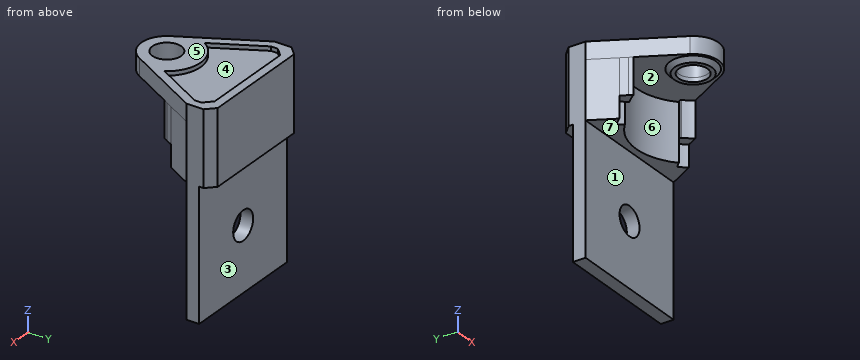
from build123d import *
from build123d.topology import SkipClean

# Parameters (mm, degrees)
BOSS_EXTRUDE1_DEPTH    = 2
BOSS_EXTRUDE2_START    = 4.75
BOSS_EXTRUDE2_DEPTH    = 4.75
BOSS_EXTRUDE3_START    = 2
SKETCH3_R              = 3
SKETCH3_R_2            = 1.7
BOSS_EXTRUDE3_DEPTH    = 2
SKETCH4_R              = 2.2
SKETCH4_R_2            = 1.7
BOSS_EXTRUDE4_DEPTH    = 0.5
CHAMFER1_SIZE          = 0.5
SKETCH5_W              = 7.5
SKETCH5_H              = 3
BOSS_EXTRUDE5_DEPTH    = 2
BOSS_EXTRUDE6_DEPTH    = 4.2
BOSS_EXTRUDE8_DEPTH    = 6.75
SKETCH10_W             = 15
SKETCH10_H             = 3
BOSS_EXTRUDE9_DEPTH    = 15.25
SKETCH11_R             = 1.65
CUT_EXTRUDE1_DEPTH     = 22.542109925
FILLET1_R              = 0.2
BOSS_EXTRUDE12_REACH   = 29.249
SKETCH16_W             = 15
SKETCH16_H             = 1.5
CUT_EXTRUDE3_DEPTH     = 0.5
CUT_EXTRUDE4_START     = -15.25
CUT_EXTRUDE4_OUTLINE_W = 15
CUT_EXTRUDE4_OUTLINE_H = 1.5
CUT_EXTRUDE4_DEPTH     = 15.25
CUT_EXTRUDE4_START_2   = -24
CUT_EXTRUDE4_2_DEPTH   = 8.75
SKETCH18_R             = 1.7
CUT_EXTRUDE5_DEPTH     = 10


# Read off the part's stored shape, not the designer's step: Cut-Extrude4
with BuildPart() as part:
    # Sketch1 → Boss-Extrude1 (new body)
    with BuildSketch(Plane.XY):
        with BuildLine():
            Line((4.594082841, 4.876925553), (5.159993549, 5.442836262))
            ThreePointArc((5.159993549, 5.442836262), (0, 7.5), (-5.159993549, 5.442836262))
            Line((-5.159993549, 5.442836262), (-4.594082841, 4.876925553))
            ThreePointArc((-4.594082841, 4.876925553), (0, 6.7), (4.594082841, 4.876925553))
        make_face()
    extrude(amount=-BOSS_EXTRUDE1_DEPTH)

    # Sketch1<3> → Boss-Extrude2 (add)
    with BuildSketch(Plane.XY.offset(BOSS_EXTRUDE2_START)):
        with BuildLine():
            Line((4.594082841, 4.876925553), (5.159993549, 5.442836262))
            ThreePointArc((5.159993549, 5.442836262), (0, 7.5), (-5.159993549, 5.442836262))
            Line((-5.159993549, 5.442836262), (-4.594082841, 4.876925553))
            ThreePointArc((-4.594082841, 4.876925553), (0, 6.7), (4.594082841, 4.876925553))
        make_face()
    extrude(amount=-BOSS_EXTRUDE2_DEPTH)

    # Sketch3 → Boss-Extrude3 (add)
    # profile 1 of 4: a face of its own
    with BuildSketch(Plane.XY.offset(4.75).offset(BOSS_EXTRUDE3_START)):
        with BuildLine():
            Line((-4.594082841, 4.876925553), (-5.159993549, 5.442836262))
            Line((-5.159993549, 5.442836262), (-2.820975701, -1.02083108))
            ThreePointArc((-2.820975701, -1.02083108), (-2.892694114, 0.795185994), (-1.902774006, 2.31936437))
            Line((-1.902774006, 2.31936437), (-2.780654635, 4.745309242))
            ThreePointArc((-2.780654635, 4.745309242), (0, 5.5), (2.780654635, 4.745309242))
            Line((2.780654635, 4.745309242), (1.902774006, 2.31936437))
            ThreePointArc((1.902774006, 2.31936437), (2.711855639, 1.282902565), (3, 0))
            ThreePointArc((3, 0), (2.954904999, -0.518205025), (2.820975701, -1.02083108))
            Line((2.820975701, -1.02083108), (5.159993549, 5.442836262))
            Line((5.159993549, 5.442836262), (4.594082841, 4.876925553))
            ThreePointArc((4.594082841, 4.876925553), (0, 6.7), (-4.594082841, 4.876925553))
        make_face()
    # profile 2 of 4: a face of its own
    with BuildSketch(Plane.XY.offset(4.75).offset(BOSS_EXTRUDE3_START)):
        with BuildLine():
            Line((-5.159993549, 5.442836262), (-4.594082841, 4.876925553))
            ThreePointArc((-4.594082841, 4.876925553), (0, 6.7), (4.594082841, 4.876925553))
            Line((4.594082841, 4.876925553), (5.159993549, 5.442836262))
            ThreePointArc((5.159993549, 5.442836262), (0, 7.5), (-5.159993549, 5.442836262))
        make_face()
    # profile 3 of 4: a face of its own
    with BuildSketch(Plane.XY.offset(4.75).offset(BOSS_EXTRUDE3_START)):
        Circle(SKETCH3_R)
        Circle(SKETCH3_R_2, mode=Mode.SUBTRACT)
    # profile 4 of 4: a face of its own
    with BuildSketch(Plane.XY.offset(4.75).offset(BOSS_EXTRUDE3_START)):
        with BuildLine():
            Line((-2.780654635, 4.745309242), (-1.902774006, 2.31936437))
            ThreePointArc((-1.902774006, 2.31936437), (0, 3), (1.902774006, 2.31936437))
            Line((1.902774006, 2.31936437), (2.780654635, 4.745309242))
            ThreePointArc((2.780654635, 4.745309242), (0, 5.5), (-2.780654635, 4.745309242))
        make_face()
    extrude(amount=-BOSS_EXTRUDE3_DEPTH)

    # Sketch4 → Boss-Extrude4 (add)
    with SkipClean():  # the faces are left unmerged after this step: merging them gives an invalid solid
        with BuildSketch(Plane(origin=(0, 0, 4.75), x_dir=(-1, 0, 0), z_dir=(0, 0, -1))):
            with Locations(Location((0, 0, 0), (0, 0, 180))):
                Circle(SKETCH4_R)
            Circle(SKETCH4_R_2, mode=Mode.SUBTRACT)
        extrude(amount=BOSS_EXTRUDE4_DEPTH)
    add(part.part.scale(1), mode=Mode.REPLACE)  # the faces are merged on a copy

    # Chamfer1
    chamfer1_edges = [part.edges().sort_by_distance(p)[0] for p in [
        (-2.2, 0, 4.75),
    ]]
    chamfer(chamfer1_edges, length=CHAMFER1_SIZE - 0.0001)  # a hair under: the kernel refuses the full size

    # Sketch5 → Boss-Extrude5 (add)
    with BuildSketch(Plane.XY.offset(6.75)):
        with BuildLine():
            ThreePointArc((-5.159993549, 5.442836262), (-2.777474396, 6.966752183), (0, 7.5))
            Line((0, 7.5), (-7.5, 7.5))
            Line((-7.5, 7.5), (-2.634698995, -1.434698995))
            ThreePointArc((-2.634698995, -1.434698995), (-2.735675101, -1.231292711), (-2.820975701, -1.02083108))
            Line((-2.820975701, -1.02083108), (-5.159993549, 5.442836262))
        make_face()
        with Locations((-3.75, 9)):
            Rectangle(SKETCH5_W, SKETCH5_H)
        with Locations((3.75, 9)):
            Rectangle(SKETCH5_W, SKETCH5_H)
        with BuildLine():
            Line((7.5, 7.5), (0, 7.5))
            ThreePointArc((0, 7.5), (2.777474396, 6.966752183), (5.159993549, 5.442836262))
            Line((5.159993549, 5.442836262), (2.820975701, -1.02083108))
            ThreePointArc((2.820975701, -1.02083108), (2.756369418, -1.184241374), (2.682306676, -1.343588812))
            Line((2.682306676, -1.343588812), (7.5, 7.5))
        make_face()
    extrude(amount=-BOSS_EXTRUDE5_DEPTH)

    # Sketch6 → Boss-Extrude6 (add)
    with SkipClean():  # the faces are left unmerged after this step: merging them gives an invalid solid
        with BuildSketch(Plane(origin=(0, 0, 4.75), x_dir=(-1, 0, 0), z_dir=(0, 0, -1))):
            with BuildLine():
                Line((-5.921621025, 4.602651891), (-5.499242594, 3.827313795))
                ThreePointArc((-5.499242594, 3.827313795), (-5.073876801, 4.375588441), (-4.594082841, 4.876925553))
                Line((-4.594082841, 4.876925553), (-5.159993549, 5.442836262))
                ThreePointArc((-5.159993549, 5.442836262), (-5.556709713, 5.037159632), (-5.921621025, 4.602651891))
            make_face()
            with BuildLine():
                Line((5.159993549, 5.442836262), (4.594082841, 4.876925553))
                ThreePointArc((4.594082841, 4.876925553), (5.074143899, 4.375278699), (5.499709828, 3.826642367))
                Line((5.499709828, 3.826642367), (5.922007367, 4.602154794))
                ThreePointArc((5.922007367, 4.602154794), (5.556921127, 5.036926403), (5.159993549, 5.442836262))
            make_face()
            with BuildLine():
                Line((-5.499242594, 3.827313795), (-5.256310338, 3.381375701))
                ThreePointArc((-5.256310338, 3.381375701), (-4.806527723, 3.994970744), (-4.285525038, 4.549370852))
                Line((-4.285525038, 4.549370852), (-4.594082841, 4.876925553))
                ThreePointArc((-4.594082841, 4.876925553), (-5.073876801, 4.375588441), (-5.499242594, 3.827313795))
            make_face()
            with BuildLine():
                Line((4.594082841, 4.876925553), (4.275732705, 4.558575417))
                ThreePointArc((4.275732705, 4.558575417), (4.802528974, 3.999776925), (5.256816116, 3.380589346))
                Line((5.256816116, 3.380589346), (5.499709828, 3.826642367))
                ThreePointArc((5.499709828, 3.826642367), (5.074143899, 4.375278699), (4.594082841, 4.876925553))
            make_face()
        extrude(amount=BOSS_EXTRUDE6_DEPTH)

    # Sketch8 → Boss-Extrude8 (add)
    with BuildSketch(Plane(origin=(0, 0, 4.75), x_dir=(-1, 0, 0), z_dir=(0, 0, -1))):
        with BuildLine():
            Line((5.922007367, 4.602154794), (7.5, 7.5))
            Line((7.5, 7.5), (7.5, 10.5))
            Line((7.5, 10.5), (-7.5, 10.5))
            Line((-7.5, 10.5), (-7.5, 7.5))
            Line((-7.5, 7.5), (-5.921621025, 4.602651891))
            ThreePointArc((-5.921621025, 4.602651891), (0.000314788, 7.499999993), (5.922007367, 4.602154794))
        make_face()
    extrude(amount=BOSS_EXTRUDE8_DEPTH)

    # Sketch10 → Boss-Extrude9 (add)
    with BuildSketch(Plane(origin=(0, 0, -2), x_dir=(-1, 0, 0), z_dir=(0, 0, -1))):
        with Locations((0, 9)):
            Rectangle(SKETCH10_W, SKETCH10_H)
    extrude(amount=BOSS_EXTRUDE9_DEPTH)

    # Sketch11 → Cut-Extrude1 (cut, through all)
    with BuildSketch(Plane.XZ.offset(-7.5)):
        with Locations(Location((0, -9.75, 0), (0, 0, 270))):
            Circle(SKETCH11_R)
    extrude(amount=-CUT_EXTRUDE1_DEPTH, mode=Mode.SUBTRACT)

    # Fillet1
    fillet1_edges = [part.edges().sort_by_distance(p)[0] for p in [
        (4.285525038, 4.549370852, 2.65),
        (-4.275732705, 4.558575417, 2.65),
    ]]
    fillet(fillet1_edges, radius=FILLET1_R)

    # Boss-Extrude12: up to this face of the body (flat: up to its plane)
    boss_extrude12_end = Plane(part.part.faces().sort_by_distance((-0.000288638, 5.532557353, 6.75))[0])
    # Sketch16 → Boss-Extrude12 (add, up to the picked face)
    with BuildSketch(Plane(origin=(0, 0, -17.25), x_dir=(-1, 0, 0), z_dir=(0, 0, -1)), mode=Mode.PRIVATE) as boss_extrude12_sk1:
        with Locations((0, 9.75)):
            Rectangle(SKETCH16_W, SKETCH16_H)
    boss_extrude12_tool1 = split(extrude(boss_extrude12_sk1.sketch, amount=-BOSS_EXTRUDE12_REACH, mode=Mode.PRIVATE), bisect_by=boss_extrude12_end, keep=Keep.BOTH, mode=Mode.PRIVATE)
    add(boss_extrude12_tool1.solids().sort_by(Axis((0, 9.75, -17.25), (0, 0, 1)))[0])

    # Sketch13 → Cut-Extrude3 (cut)
    with BuildSketch(Plane.XY.offset(6.75)):
        with BuildLine():
            ThreePointArc((3.4124071, 2.086978147), (-0.000677338, 3.999999943), (-3.413113698, 2.085822351))
            Line((-3.413113698, 2.085822351), (-6.5, 7.754618569))
            Line((-6.5, 7.754618569), (-6.5, 8.585786438))
            Line((-6.5, 8.585786438), (-5.585786438, 9.5))
            Line((-5.585786438, 9.5), (5.585786438, 9.5))
            Line((5.585786438, 9.5), (6.5, 8.585786438))
            Line((6.5, 8.585786438), (6.5, 7.754711685))
            Line((6.5, 7.754711685), (3.4124071, 2.086978147))
        make_face()
    extrude(amount=-CUT_EXTRUDE3_DEPTH, mode=Mode.SUBTRACT)

    # Cut-Extrude4 outline → Cut-Extrude4 (cut)
    with BuildSketch(Plane(origin=(0, 0, -17.25), x_dir=(-1, 0, 0), z_dir=(0, 0, -1)).offset(CUT_EXTRUDE4_START)):
        with Locations((0, 9.75)):
            Rectangle(CUT_EXTRUDE4_OUTLINE_W, CUT_EXTRUDE4_OUTLINE_H)
    extrude(amount=CUT_EXTRUDE4_DEPTH, mode=Mode.SUBTRACT)

    # Cut-Extrude4 2 outline → Cut-Extrude4 2 (cut)
    with BuildSketch(Plane(origin=(0, 0, -17.25), x_dir=(-1, 0, 0), z_dir=(0, 0, -1)).offset(CUT_EXTRUDE4_START_2)):
        Polygon((-7.5, 10.5), (-7.5, 9.5), (-6.5, 10.5), align=None)
        Polygon((7.5, 10.5), (6.5, 10.5), (7.5, 9.5), align=None)
    extrude(amount=CUT_EXTRUDE4_2_DEPTH, mode=Mode.SUBTRACT)

    # Sketch18 → Cut-Extrude5 (cut)
    with BuildSketch(Plane(origin=(0, 10.5, 0), x_dir=(1, 0, 0), z_dir=(0, 1, 0))):
        with Locations(Location((0, 9.75, 0), (0, 0, 90))):
            Circle(SKETCH18_R)
    extrude(amount=-CUT_EXTRUDE5_DEPTH, mode=Mode.SUBTRACT)


solid = part.part
The listing builds one solid part. Answer for the finished solid, in the listing's coordinates (mm). Face numbers are marked on the shaded views. A direction names the side the tool comes from. Coordinates: 2 decimals unless noted, no trailing zeros. Loops run counter-clockwise (first coordinate to the right, second up) from the corner with the lowest first, then second, coordinate; pieces in that order, holes last.
1) Determine the mould class of the marked faces 5, 6 and 7 for opening direction Z: pulls with the +Z half, pulls with the -Z half, needs draft (parallel to the pull), parting line crosses it, or undercut.
2) Find section A-A on z = -9.75. Write down the section's boundary in (x, y).
3) Find section B-B on x = 0. Give the number of separate pieces and of enclosed holes in the cut face, then the cut area to 3 significant figures.
4) Find the intervals of material crossed by L1, parallel to Y at x = 0, z = 6.3; L2, parallel to Y at x = 0, z = 5.4; L3, parallel to Z at x = -1.5, y = 5.5, in increasing order.
5) Find section D-D on z = -0.5. Write down the section's boundary in (x, y).
6) A tool of negligible diameter and unlimited length cuts with its end or side. For the marked faces 1, 2, 3 and 4, from which of +Z, -Z, +X, -X, +Y, -Y can it reach the whole face along a straight path? Write none if from no direction.
7) Flat-ended cylindrical pins translate along their axes: pin 1 Ø5 at (x, z) = (-4.5, -7) entering from +Y; pin 2 Ø3.5 at (x, y) = (1, 6.5) entering from +Z; pin 3 Ø4.5 at (x, y) = (0, 0) entering from -Z. Find the tip coordinate at first contact, or state that the pin passes through.
Values:
1. face 5: pulls with the +Z half
1. face 6: needs draft
1. face 7: pulls with the -Z half
2. outline: (-7.5, 7.5) - (-1.7, 7.5) - (-1.7, 9) - (-7.5, 9) - close; (1.7, 7.5) - (7.5, 7.5) - (7.5, 9) - (1.7, 9) - close
3. separate pieces: 3
3. enclosed holes: 0
3. area: 61.6 mm2
4. L1: y = -3 to -1.7, 1.7 to 4, 9.5 to 10.5
4. L2: y = -3 to -1.7, 1.7 to 10.5
4. L3: z = 4.75 to 6.25
5. outline: (-7.5, 7.5) - (-5.92, 4.6) arc R7.5 cw to (-5.16, 5.44) - (-4.59, 4.88) arc R6.7 cw to (4.59, 4.88) - (5.16, 5.44) arc R7.5 cw to (5.92, 4.6) - (7.5, 7.5) - (7.5, 9.5) - (6.5, 10.5) - (-6.5, 10.5) - (-7.5, 9.5) - close
6. face 1: -Z, +X, -X, -Y
6. face 2: -Z
6. face 3: -Z, +X, -X, +Y
6. face 4: +Z
7. pin 1: stops at y = 9
7. pin 2: stops at z = 6.25
7. pin 3: stops at z = 4.25
